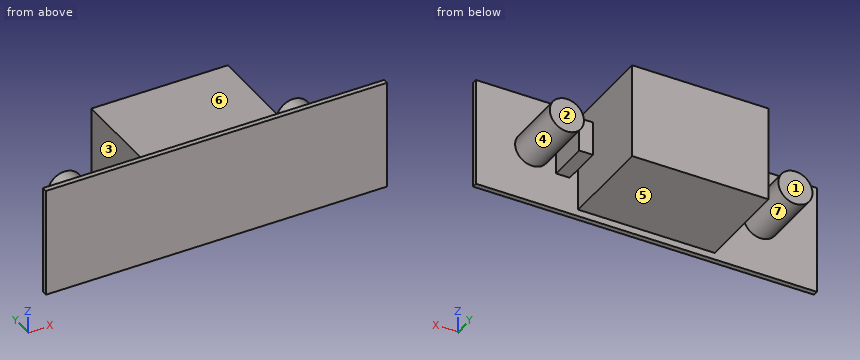
```python
from build123d import *

# Parameters (mm, degrees)
SKETCH_1_W      = 100
SKETCH_1_H      = 32
EXTRUDE_1_DEPTH = 1.5
SKETCH_2_W      = 40
SKETCH_2_H      = 28
EXTRUDE_2_DEPTH = 28
SKETCH_3_R      = 5
EXTRUDE_3_DEPTH = 18
SKETCH_4_W      = 4
SKETCH_4_H      = 10
EXTRUDE_4_DEPTH = 12


with BuildPart() as part:
    # 草图1 → 凸台-拉伸1 (new body)
    with BuildSketch(Plane(origin=(0, 0, 0), x_dir=(1, 0, 0), z_dir=(0, 1, 0))):
        with Locations((50, 16)):
            Rectangle(SKETCH_1_W, SKETCH_1_H)
    extrude(amount=EXTRUDE_1_DEPTH)

    # 草图2 → 凸台-拉伸2 (add)
    with BuildSketch(Plane(origin=(0, 1.5, 0), x_dir=(1, 0, 0), z_dir=(0, 1, 0))):
        with Locations((50, 16.000816198)):
            Rectangle(SKETCH_2_W, SKETCH_2_H)
    extrude(amount=EXTRUDE_2_DEPTH)

    # 草图3 → 凸台-拉伸3 (add)
    with BuildSketch(Plane(origin=(0, 1.5, 0), x_dir=(1, 0, 0), z_dir=(0, 1, 0))):
        with Locations(Location((16.5, 16, 0), (0, 0, 90))):
            Circle(SKETCH_3_R)
        with Locations(Location((83.5, 16, 0), (0, 0, 90))):
            Circle(SKETCH_3_R)
    extrude(amount=EXTRUDE_3_DEPTH)

    # 草图4 → 凸台-拉伸4 (add)
    with BuildSketch(Plane(origin=(0, 1.5, 0), x_dir=(1, 0, 0), z_dir=(0, 1, 0))):
        with Locations((74.5, 16)):
            Rectangle(SKETCH_4_W, SKETCH_4_H)
    extrude(amount=EXTRUDE_4_DEPTH)


solid = part.part
```
Here's how the part is built. I have some questions about the finished solid (model axes, mm). Face numbers are marked on the shaded views. A direction names the side the tool comes from. Coordinates: 2 decimals unless noted, no trailing zeros. Write each loop counter-clockwise with the first axis right and the second up, starting at its lowest first coordinate (ties: lowest second). Pieces come first, ordered by that corner, then holes. Notation, with made-up numbers: (-1.75, 60) -> (38.25, 60) arc R27 ccw to (38.25, 88) -> close; hole circle Ø7 at (34, 61). An arc over 180 degrees is marked (long way). Use a Markdown table: item, result. Add a question column.
(1) If we section it at A-A, the plane y = 9: Write out the boundary of the cut face in (x, z).
(2) We'd pull the mould along X, two halves only. Please class the marked faces 6 and 7: +X half, -X half, draft (parallel to the pull), parting line (faces both ways), or undercut.
(3) If we section it at C-C, the plane z = -27: Write out the boundary of the cut face in (x, y).
(4) If we section it at D-D, the plane y = 27.5: Write out the boundary of the cut face in (x, z), and give its area (3 significant figures).
(5) I'm going to push flat-ended pins straight in: P1, Ø11, axis at x = 85.5, z = -14, coming from the +Y side; P2, Ø14, axis at y = 21, z = -19, coming from the +X side; P3, Ø8.5, axis at x = 47.5, y = 16.5, coming from the -Z side. Where does each tip first touch, or does it pass through?
(6) If we section it at B-B, the plane x = 57: Write out the boundary of the cut face in (y, z), and give its area (3 significant figures).
(7) Please list where these lines run through material, in increasing order: line 1 (X direction, y = 3, z = -17); line 2 (X direction, y = 10.75, z = -20); line 3 (Y direction, x = 19, z = -29.5).
(8) For the marked faces 1, 2, 3, 4 and 5, which set-ups out of +Z, -Z, +X, -X, +Y, -Y let a thin tool reach every point of the face, with its end or its side?
Outcome:
| question | item | result |
|---|---|---|
| 1 | outline | circle Ø10 at (16.5, -16); (30, -30) -> (70, -30) -> (70, -2) -> (30, -2) -> close; (72.5, -21) -> (76.5, -21) -> (76.5, -11) -> (72.5, -11) -> close; circle Ø10 at (83.5, -16) |
| 2 | face 6 | draft |
| 2 | face 7 | undercut |
| 3 | outline | (0, 0) -> (100, 0) -> (100, 1.5) -> (70, 1.5) -> (70, 29.5) -> (30, 29.5) -> (30, 1.5) -> (0, 1.5) -> close |
| 4 | outline | (30, -30) -> (70, -30) -> (70, -2) -> (30, -2) -> close |
| 4 | area | 1,120 mm^2 |
| 5 | P1 | stops at y = 19.5 |
| 5 | P2 | stops at x = 88.5 |
| 5 | P3 | stops at z = -30 |
| 6 | outline | (0, -32) -> (1.5, -32) -> (1.5, -30) -> (29.5, -30) -> (29.5, -2) -> (1.5, -2) -> (1.5, 0) -> (0, 0) -> close |
| 6 | area | 832 mm^2 |
| 7 | line 1 | x = 11.6 to 21.4, 30 to 70, 72.5 to 76.5, 78.6 to 88.4 |
| 7 | line 2 | x = 13.5 to 19.5, 30 to 70, 72.5 to 76.5, 80.5 to 86.5 |
| 7 | line 3 | y = 0 to 1.5 |
| 8 | face 1 | +Z, -Z, -X, +Y |
| 8 | face 2 | +Z, -Z, +X, +Y |
| 8 | face 3 | +Z, -Z, +Y |
| 8 | face 4 | +Y |
| 8 | face 5 | -Z, +X, -X, +Y |
